The model under review builds one solid part; all positions refer to its coordinate system, in mm. A direction names the side the tool comes from. Round coordinates to 2 decimals unless told otherwise and drop trailing zeros. Write each loop counter-clockwise with the first axis right and the second up, starting at its lowest first coordinate (ties: lowest second). Pieces come first, ordered by that corner, then holes. Notation, with made-up numbers: (55.25, -3) -> (98.25, -3) arc R3 cw to (98.25, 1) -> close; hole circle Ø5 at (41, -7). An arc over 180 degrees is marked (long way). Return JSON: item names as keys, results as strings. Group by question number.
1. Take a section at C-C, the plane y = 38. Write out the cut boundary in (x, z).
2. Tool access review of faces 1 (the flat face through (5, -9, 3)), 2 (the flat face through (3.228, -6, 2)), 3 (the flat face through (-2, 29, 3)): name each direction out of +Z, -Z, +X, -X, +Y, -Y from which nothing blocks a thin tool from reaching the whole face with its end or side.
3. For line 1 along Y through (x, z) = (-12.5, 3.75); line 2 along Y through (x, z) = (-8, 1.85); line 3 along X through (y, z) = (68, 1.2), list the stretches that pass through material, from the lowest coordinate up. Write a range as from..to.
4. Clearance check with flat-ended pins moving along their axes: P1, Ø7, axis at x = -1.5, y = 19.5, coming from the +Z side; P2, Ø1.1, axis at x = 5, z = 3.5, coming from the -Y side; P3, Ø1.5, axis at x = -19.5, z = 2, coming from the -Y side; P4, Ø1.5, axis at x = -22, z = 1, coming from the -Y side. State where each tip first meets the part, or that it passes through.
5. Take a section at D-D, the plane y = 57. Write out the cut boundary in (x, z), then the cut area to 3 significant figures.
6. Mouldability with a two-part tool opening along Y and no side actions: class faces 4 (the flat face through (-24.132, 74, 2)), 5 (the flat face through (-5, 19.289, 1)), 6 (the flat face through (3, 9, 3)) as pulls with the +Y half, pulls with the -Y half, needs draft (parallel to the pull), parting line crosses it, or undercut.
7. Take a section at A-A, the plane z = 1.65. Write out the cut boundary in (x, y), then the cut area to 3 significant figures.
from build123d import *

# Parameters (mm, degrees)
BOSS_EXTRUDE2_DEPTH = 3
SKETCH2_W           = 34.2
SKETCH2_H           = 1
SKETCH2_W_2         = 30.78
SKETCH2_W_3         = 27.36
SKETCH2_W_4         = 23.94
SKETCH2_W_5         = 20.52
SKETCH2_W_6         = 17.1
SKETCH2_W_7         = 13.68
SKETCH2_W_8         = 10.26
SKETCH2_W_9         = 6.84
SKETCH2_W_10        = 3.42
BOSS_EXTRUDE3_DEPTH = 1


with BuildPart() as part:
    # Sketch1 → Boss-Extrude2 (new body)
    with BuildSketch(Plane.XY):
        Polygon((-27.552134831, 89.289101124), (-24.132134831, 89.289101124), (-20.712134831, 89.289101124), (-17.292134831, 89.289101124), (-13.872134831, 89.289101124), (-10.452134831, 89.289101124), (-7.032134831, 89.289101124), (-3.612134831, 89.289101124), (-0.192134831, 89.289101124), (3.227865169, 89.289101124), (6.647865169, 89.289101124), (6.647865169, 79.289101124), (6.647865169, 69.289101124), (6.647865169, 59.289101124), (6.647865169, 49.289101124), (6.647865169, 39.289101124), (6.647865169, 29.289101124), (6.647865169, 19.289101124), (6.647865169, 9.289101124), (6.647865169, -0.710898876), (6.647865169, -10.710898876), (3.227865169, -10.710898876), (3.227865169, -0.710898876), (-0.192134831, -0.710898876), (-0.192134831, 9.289101124), (-3.612134831, 9.289101124), (-3.612134831, 19.289101124), (-7.032134831, 19.289101124), (-7.032134831, 29.289101124), (-10.452134831, 29.289101124), (-10.452134831, 39.289101124), (-13.872134831, 39.289101124), (-13.872134831, 49.289101124), (-17.292134831, 49.289101124), (-17.292134831, 59.289101124), (-20.712134831, 59.289101124), (-20.712134831, 69.289101124), (-24.132134831, 69.289101124), (-24.132134831, 79.289101124), (-27.552134831, 79.289101124), align=None)
    extrude(amount=BOSS_EXTRUDE2_DEPTH)

    # Sketch2 → Boss-Extrude3 (add)
    with BuildSketch(Plane.XY.offset(3)):
        with Locations((-10.452134831, 83.789101124)):
            Rectangle(SKETCH2_W, SKETCH2_H)
        with Locations((-8.742134831, 73.789101124)):
            Rectangle(SKETCH2_W_2, SKETCH2_H)
        with Locations((-7.032134831, 63.789101124)):
            Rectangle(SKETCH2_W_3, SKETCH2_H)
        with Locations((-5.322134831, 53.789101124)):
            Rectangle(SKETCH2_W_4, SKETCH2_H)
        with Locations((-3.612134831, 43.789101124)):
            Rectangle(SKETCH2_W_5, SKETCH2_H)
        with Locations((-1.902134831, 33.789101124)):
            Rectangle(SKETCH2_W_6, SKETCH2_H)
        with Locations((-0.192134831, 23.789101124)):
            Rectangle(SKETCH2_W_7, SKETCH2_H)
        with Locations((1.517865169, 13.789101124)):
            Rectangle(SKETCH2_W_8, SKETCH2_H)
        with Locations((3.227865169, 3.789101124)):
            Rectangle(SKETCH2_W_9, SKETCH2_H)
        with Locations((4.937865169, -6.210898876)):
            Rectangle(SKETCH2_W_10, SKETCH2_H)
    extrude(amount=BOSS_EXTRUDE3_DEPTH)


solid = part.part
Output:
{
 "1": {"outline": "(-10.45, 0) -> (6.65, 0) -> (6.65, 3) -> (-10.45, 3) -> close"},
 "2": {"face 1": "+Z, +X, -X, -Y", "face 2": "+Z, -Z, -X, -Y", "face 3": "+Z, +X, -X"},
 "3": {"line 1": "y = 43.29..44.29, 53.29..54.29, 63.29..64.29, 73.29..74.29, 83.29..84.29", "line 2": "y = 29.29..89.29", "line 3": "x = -20.71..6.65"},
 "4": {"P1": "stops at z = 3", "P2": "stops at y = -10.71", "P3": "stops at y = 59.29", "P4": "stops at y = 69.29"},
 "5": {"outline": "(-17.29, 0) -> (6.65, 0) -> (6.65, 3) -> (-17.29, 3) -> close", "area": "71.8 mm^2"},
 "6": {"face 4": "needs draft", "face 5": "pulls with the -Y half", "face 6": "undercut"},
 "7": {"outline": "(-27.55, 79.29) -> (-24.13, 79.29) -> (-24.13, 69.29) -> (-20.71, 69.29) -> (-20.71, 59.29) -> (-17.29, 59.29) -> (-17.29, 49.29) -> (-13.87, 49.29) -> (-13.87, 39.29) -> (-10.45, 39.29) -> (-10.45, 29.29) -> (-7.03, 29.29) -> (-7.03, 19.29) -> (-3.61, 19.29) -> (-3.61, 9.29) -> (-0.19, 9.29) -> (-0.19, -0.71) -> (3.23, -0.71) -> (3.23, -10.71) -> (6.65, -10.71) -> (6.65, 89.29) -> (-27.55, 89.29) -> close", "area": "1,880 mm^2"}
}
